Read the model definition and answer for the solid it produces. Units are mm, in the model's axes. Face numbers are marked on the shaded views. Round coordinates to 2 decimals unless told otherwise and drop trailing zeros. Write each loop counter-clockwise with the first axis right and the second up, starting at its lowest first coordinate (ties: lowest second). Pieces come first, ordered by that corner, then holes.
from build123d import *

# Parameters (mm, degrees)
BASE_DEPTH              = 4.1656
F_3_8_16_TAPPED_HOLE1_D = 7.9375


with BuildPart() as part:
    # Sketch1 → BASE (new, symmetric)
    with BuildSketch(Plane(origin=(0, 0, 0), x_dir=(0, 0, -1), z_dir=(1, 0, 0))):
        Polygon((0, 8.182900835), (-7.0866, 4.091450418), (-7.0866, -4.091450418), (0, -8.182900835), (7.0866, -4.091450418), (7.0866, 4.091450418), align=None)
    extrude(amount=BASE_DEPTH, both=True)

    # Sketch2 → EDGE-CUT (revolve, cut)
    with BuildSketch(Plane.XY, mode=Mode.PRIVATE) as edge_cut_sk:
        Polygon((4.1656, 6.912900835), (3.49291061, 8.182900835), (4.1656, 8.182900835), align=None)
    edge_cut = revolve(edge_cut_sk.sketch.rotate(Axis((0, 0, 0), (1, 0, 0)), 90), axis=Axis((0, 0, 0), (1, 0, 0)), mode=Mode.SUBTRACT)

    # Mirror1: EDGE-CUT across plane
    add(edge_cut.mirror(Plane(origin=(0, 0, 0), x_dir=(0, 0, 1), z_dir=(1, 0, 0))), mode=Mode.SUBTRACT)

    # 3/8-16 Tapped Hole1 (through all)
    with Locations(Plane(origin=(4.1656, 0, 0), x_dir=(0, 0, -1), z_dir=(1, 0, 0))):
        with Locations((0, 0)):
            Hole(F_3_8_16_TAPPED_HOLE1_D / 2)


solid = part.part
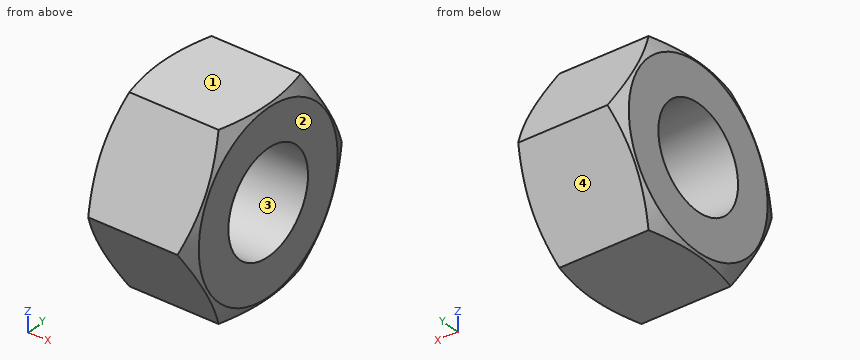
Q1. Section B-B (x = -2) is taken. Determine the outline of the cut face in (y, z), then the cut area to 3 significant figures.
Verdict:
outline: (-8.18, 0) - (-4.09, -7.09) - (4.09, -7.09) - (8.18, 0) - (4.09, 7.09) - (-4.09, 7.09) - close; hole circle Ø7.94 at (0, 0)
area: 124 mm2
Q2. Section A-A (y = 0) is taken. Determine the outline of the cut face in (x, z).
Verdict:
outline: (-4.17, -6.91) - (-4.07, -7.09) - (4.07, -7.09) - (4.17, -6.91) - (4.17, -3.97) - (-4.17, -3.97) - close; (-4.17, 3.97) - (4.17, 3.97) - (4.17, 6.91) - (4.07, 7.09) - (-4.07, 7.09) - (-4.17, 6.91) - close
Q3. A flat-ended cylindrical pin translates along its axis: pin 1 Ø3 at (x, z) = (2.5, -4) entering from -Y. Find the tip coordinate at first contact, or state that the pin passes through.
Verdict:
pin 1: stops at y = -6.74
Q4. Determine the mould class of the marked faces 1, 2, 3 and 4 for opening direction Z: pulls with the +Z half, pulls with the -Z half, needs draft (parallel to the pull), parting line crosses it, or undercut.
Verdict:
face 1: pulls with the +Z half
face 2: needs draft
face 3: undercut
face 4: pulls with the -Z half
Q5. Straight lines are drawn through the part: probe 1 along Y at (x, z) = (2.5, 2.5); probe 2 along Y at (x, z) = (-3.5, -3.5); probe 3 along Z at (x, y) = (1, 1.75). For each, find the intervals that lie inside material, in ascending order.
Verdict:
probe 1: y = -6.74 to -3.08, 3.08 to 6.74
probe 2: y = -6.16 to -1.87, 1.87 to 6.16
probe 3: z = -7.09 to -3.56, 3.56 to 7.09
